Source: CAD feature listing. Evaluate the final solid. Frame: model axes, mm. Face numbers are marked on the shaded views. Coordinates: 2 decimals unless noted, no trailing zeros. Order: outer loops, then holes, each group sorted by start corner. A loop starts at its lowest first (then second) coordinate and runs counter-clockwise, first axis right, second up.
```python
from build123d import *

# Parameters (mm, degrees)
F0_R     = 1.016
F1_DEPTH = 2.2225
F2_R     = 2.54
F3_R     = 2.54


# Not quite as in the source:
# - a length typed as a fraction of an inch, garbled in the dataset ("3 / 203.2 mm" for 3/8 in), is restored


with BuildPart() as f1:
    # F0 (on Front) → F1 (new body)
    with BuildSketch(Plane.XZ):
        with BuildLine():
            Line((3.2593966339, 1.5410604233), (0, 2.794))
            ThreePointArc((0, 2.794), (-2.794, 0), (0, -2.794))
            Line((0, -2.794), (3.2593966339, -1.5410604233))
            ThreePointArc((3.2593966339, -1.5410604233), (4.318, 0), (3.2593966339, 1.5410604233))
        make_face()
        Circle(F0_R, mode=Mode.SUBTRACT)
    extrude(amount=F1_DEPTH)

    # F2
    f2_edges = [f1.edges().sort_by_distance(p)[0] for p in [
        (0, -1.11125, 2.794),
    ]]
    fillet(f2_edges, radius=F2_R)

    # F3
    f3_edges = [f1.edges().sort_by_distance(p)[0] for p in [
        (0, -1.11125, -2.794),
    ]]
    fillet(f3_edges, radius=F3_R)


solid = f1.part
```
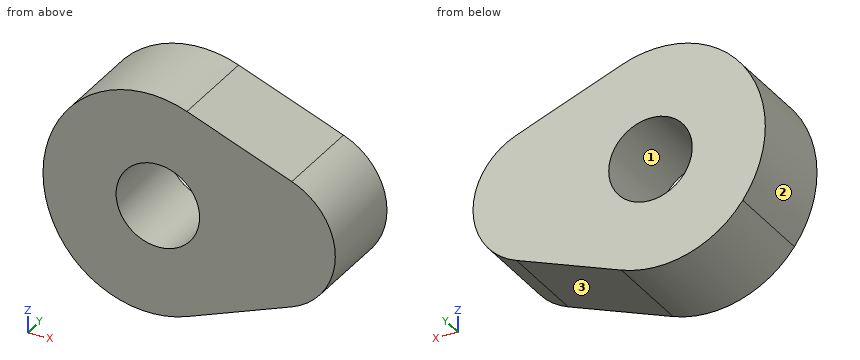
1. Ray query, line 1 (Z direction, x = -0.25, y = -2.05); line 2 (X direction, y = -0.8, z = 0.55); line 3 (X direction, y = -0.25, z = 0.7). Return the intervals inside material, ascending.
Findings:
line 1: z = -2.69 to -0.98, 0.98 to 2.69
line 2: x = -2.74 to -0.85, 0.85 to 4.22
line 3: x = -2.7 to -0.74, 0.74 to 4.16
2. Section query A-A on z = 0. Return loops of the section in (x, y).
Findings:
outline: (-2.79, -2.22) - (-1.02, -2.22) - (-1.02, 0) - (-2.79, 0) - close; (1.02, -2.22) - (4.32, -2.22) - (4.32, 0) - (1.02, 0) - close
3. Draft query along X for the marked faces 1, 2 and 3. Return one class per face: released by +X, released by -X, zero draft, split by the parting line, or undercut.
Findings:
face 1: undercut
face 2: released by -X
face 3: released by +X
4. Section query C-C on y = -0.45. Return loops of the section in (x, z), plus the area to 3 significant figures.
Findings:
outline: (-2.24, -1.66) arc R2.54 ccw to (0.71, -2.52) - (3.26, -1.54) arc R1.65 ccw to (3.26, 1.54) - (0.71, 2.52) arc R2.54 ccw to (-2.24, 1.66) arc R2.79 ccw to start; hole circle Ø2.03 at (0, 0)
area: 25.3 mm2
5. Section query B-B on x = 0. Return loops of the section in (y, z).
Findings:
outline: (-2.22, -2.68) - (0, -2.68) - (0, -1.02) - (-2.22, -1.02) - close; (-2.22, 1.02) - (0, 1.02) - (0, 2.68) - (-2.22, 2.68) - close
6. Section query D-D on x = 2.5. Return loops of the section in (y, z).
Findings:
outline: (-2.22, -1.83) - (0, -1.83) - (0, 1.83) - (-2.22, 1.83) - close
